Autodesk Inventor part; units mm, degrees
ref_plane "YZ Plane" through (0, 0, 0) normal (1, 0, 0) x (0, 1, 0)
ref_plane "XZ Plane" through (0, 0, 0) normal (0, 1, 0) x (-1, 0, 0)
ref_plane "XY Plane" through (0, 0, 0) normal (0, 0, 1) x (1, 0, 0)
sketch "Sketch1" plane through (0, 0, 0) normal (0, 0, 1) x (1, 0, 0)
  line L0 (-20, 10) -> (20, 10)
  line L1 (20, 10) -> (20, -10)
  line L2 (20, -10) -> (-20, -10)
  line L3 (-20, -10) -> (-20, 10)
  line L4 (-20, 10) -> (20, -10) construction
  line L5 (20, 10) -> (-20, -10) construction
  line L6 (18, 8) -> (-18, 8)
  line L7 (-18, 8) -> (-18, -8)
  line L8 (-18, -8) -> (18, -8)
  line L9 (18, -8) -> (18, 8)
  point P0 (0, 0)
  dimension "d0" = 40
  dimension "d1" = 20
  dimension "d2" = 2
extrude "Extrusion1" add sketch "Sketch1" along normal mid plane 263
fillet "Fillet1" radius 2 4 edges at (-20, 10, 0) (-20, -10, 0) (20, -10, 0) (20, 10, 0)
sketch "Sketch4" plane through (0, 0, 0) normal (0, 1, 0) x (-1, 0, 0)
  line L0 (18, 131.5) -> (-18, 131.5)
  line L1 (-18, -131.5) -> (18, -131.5)
  circle A0 centre (0, 116.5) radius 4.5
  circle A1 centre (0, -116.5) radius 4.5
  line L2 (48.8004, 0) -> (-48.8004, 0) construction
  point P0 (0, 0)
  point P1 (0, 0)
  dimension "d20" = 9
  dimension "d21" = 15
extrude "Extrusion4" cut sketch "Sketch4" along normal through all both and the other way through all
properties part number "Leg tube 2"
Part model, mm, in its own coordinate system. A direction names the side the tool comes from. Round coordinates to 2 decimals unless told otherwise and drop trailing zeros. Loops run counter-clockwise (first coordinate to the right, second up) from the corner with the lowest first, then second, coordinate; pieces in that order, holes last. Notation, with made-up numbers: (53.5, -20) - (110.5, -20) arc R21 cw to (110.5, 3) - close; hole circle Ø4 at (67.5, 78.5). An arc over 180 degrees is marked (long way). Answer as a JSON object with one key per item and string values.
Item 1: Pull direction Z, two halves, no side cores. Call faces 3 (the face through (0, 8, -2)), 4 (the face through (3.6, -9, -119.2)), 5 (the face through (-1.6, 8.2, -131.5)), 6 (the face through (3.6, -9, 113.8)): pulls with the +Z half, pulls with the -Z half, needs draft (parallel to the pull), parting line crosses it, or undercut.
Output:
{"face 3": "needs draft", "face 4": "undercut", "face 5": "pulls with the -Z half", "face 6": "undercut"}
Item 2: Band-saw the part on A-A on x = 0. List the corners of the cut face in (y, z), plus the area to 3 significant figures.
Output:
{"outline": "(-10, -131.5) - (-8, -131.5) - (-8, -121) - (-10, -121) - close; (-10, -112) - (-8, -112) - (-8, 112) - (-10, 112) - close; (-10, 121) - (-8, 121) - (-8, 131.5) - (-10, 131.5) - close; (8, -131.5) - (10, -131.5) - (10, -121) - (8, -121) - close; (8, -112) - (10, -112) - (10, 112) - (8, 112) - close; (8, 121) - (10, 121) - (10, 131.5) - (8, 131.5) - close", "area": "980 mm2"}
Item 3: Band-saw the part on D-D on x = 14. List the corners of the cut face in (y, z), plus the area to 3 significant figures.
Output:
{"outline": "(-10, -131.5) - (-8, -131.5) - (-8, 131.5) - (-10, 131.5) - close; (8, -131.5) - (10, -131.5) - (10, 131.5) - (8, 131.5) - close", "area": "1,050 mm2"}
Item 4: Band-saw the part on B-B on y = -1.25. List the corners of the cut face in (x, z), plus the area to 3 significant figures.
Output:
{"outline": "(-20, -131.5) - (-18, -131.5) - (-18, 131.5) - (-20, 131.5) - close; (18, -131.5) - (20, -131.5) - (20, 131.5) - (18, 131.5) - close", "area": "1,050 mm2"}
Item 5: Wall check: L1, parallel to Z at x = 0, y = -8.7; L2, parallel to X at y = 6.5, z = -64; L3, parallel to Y at x = 1, z = -20. Give the ranges that are in metal, low to high.
Output:
{"L1": "-131.5 to -121, -112 to 112, 121 to 131.5", "L2": "-20 to -18, 18 to 20", "L3": "-10 to -8, 8 to 10"}
Item 6: Band-saw the part on C-C on z = 116.5. List the corners of the cut face in (x, y).
Output:
{"outline": "(-20, -8) arc R2 ccw to (-18, -10) - (-4.5, -10) - (-4.5, -8) - (-18, -8) - (-18, 8) - (-4.5, 8) - (-4.5, 10) - (-18, 10) arc R2 ccw to (-20, 8) - close; (4.5, -10) - (18, -10) arc R2 ccw to (20, -8) - (20, 8) arc R2 ccw to (18, 10) - (4.5, 10) - (4.5, 8) - (18, 8) - (18, -8) - (4.5, -8) - close"}
Item 7: Pin check, flat tip, straight feed: pin 1 (7 mm diameter, centred on x = 0, z = -116.5, fed in from +Y) (3 decimals). Stop position of the tip, or through.
Output:
{"pin 1": "through"}
Item 8: Tool access for faces 1 (the face through (-20, 0, -2)), 2 (the face through (0, -8, -2)): list every direction of +Z, -Z, +X, -X, +Y, -Y with a clear straight run to the whole face (end or side of a thin tool).
Output:
{"face 1": "+Z, -Z, -X, +Y, -Y", "face 2": "+Z, -Z"}
